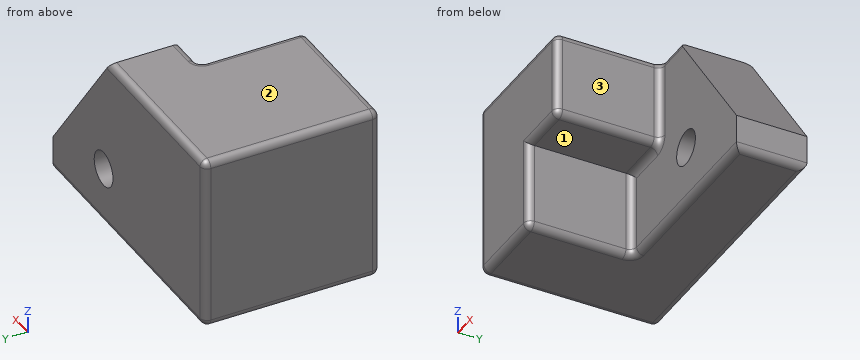
from build123d import *

# Parameters (mm, degrees)
F0_W     = 203.2
F0_H     = 127
F1_DEPTH = 127
F3_DEPTH = 76.2
F4_SIZE2 = 101.6
F4_SIZE  = 76.2
F5_R     = 5.08
F6_R     = 12.6476198181
F7_DEPTH = 78.486


with BuildPart() as f1:
    # F0 (on Front) → F1 (new body)
    with BuildSketch(Plane.XZ):
        Rectangle(F0_W, F0_H)
    extrude(amount=F1_DEPTH)

    # F2 (on face) → F3 (cut)
    with BuildSketch(Plane.XZ.offset(127)):
        Polygon((101.6, 63.5), (0, 63.5), (0, 0), (-38.1, 0), (-38.1, -63.5), (101.6, -63.5), align=None)
    extrude(amount=-F3_DEPTH, mode=Mode.SUBTRACT)

    # F4
    f4_edges = [f1.edges().sort_by_distance(p)[0] for p in [
        (101.6, -25.4, 63.5),
    ]]
    f4_side = f1.faces().sort_by_distance((-21.771429, -52.614286, 63.5))[0]
    chamfer(f4_edges, length=F4_SIZE, length2=F4_SIZE2, reference=f4_side)

    # F5
    f5_edges = [f1.edges().sort_by_distance(p)[0] for p in [
        (0, -88.9, 63.5),
        (-50.8, -127, 63.5),
        (-19.05, -127, 0),
        (0, -127, 31.75),
        (0, -88.9, 0),
        (-38.1, -127, -31.75),
        (-38.1, -88.9, -63.5),
        (-69.85, -127, -63.5),
        (0, -50.8, 31.75),
        (31.75, -50.8, -63.5),
        (-38.1, -50.8, -31.75),
        (0, 0, -63.5),
        (-38.1, 0, 63.5),
        (-101.6, -127, 0),
        (-101.6, -63.5, 63.5),
        (-101.6, 0, 0),
        (101.6, -25.4, -63.5),
        (-101.6, -63.5, -63.5),
        (12.7, -50.8, 63.5),
        (-19.05, -50.8, 0),
    ]]
    fillet(f5_edges, radius=F5_R)

    # F6 (on face) → F7 (cut)
    with BuildSketch(Plane.XZ.offset(50.8)):
        with Locations((33.5065871477, -21.8299999833)):
            Circle(F6_R)
    extrude(amount=-F7_DEPTH, mode=Mode.SUBTRACT)


solid = f1.part
Geometry check sheet. Reference: the model listing, model coordinates, mm. Face numbers are marked on the shaded views. A direction names the side the tool comes from. Round coordinates to 2 decimals unless told otherwise and drop trailing zeros. Write each loop counter-clockwise with the first axis right and the second up, starting at its lowest first coordinate (ties: lowest second). Pieces come first, ordered by that corner, then holes.
Item 1: Go/stop test with flat-tipped pins: pin 1 Ø12 at (x, z) = (80.5, -6) entering from -Y; pin 2 Ø4 at (y, z) = (-111.5, -13.5) entering from +X. Record where each tip stops, or that it passes through.
Determined:
pin 1: stops at y = -50.8
pin 2: stops at x = -38.1
Item 2: Section check C-C (y = -82). Record the boundary of the cut face in (x, z), plus the area to 3 significant figures.
Determined:
outline: (-101.6, -58.42) arc R5.08 ccw to (-96.52, -63.5) - (-43.18, -63.5) arc R5.08 ccw to (-38.1, -58.42) - (-38.1, 0) - (-5.08, 0) arc R5.08 ccw to (0, 5.08) - (0, 58.42) arc R5.08 ccw to (-5.08, 63.5) - (-96.52, 63.5) arc R5.08 ccw to (-101.6, 58.42) - close
area: 10,500 mm2
Item 3: Access from +Z, -Z, +X, -X, +Y, -Y to the whole of each face (thin tool, end or side, straight path). Record for the marked faces 1, 2 and 3.
Determined:
face 1: -Z, +X, -Y
face 2: +Z, +X, -X, +Y, -Y
face 3: +Z, -Z, +X, -Y
Item 4: Section check A-A (y = -27.5). Record the boundary of the cut face in (x, z).
Determined:
outline: (-101.6, -58.42) arc R5.08 ccw to (-96.52, -63.5) - (96.52, -63.5) arc R5.08 ccw to (101.6, -58.42) - (101.6, -38.1) - (25.4, 63.5) - (-96.52, 63.5) arc R5.08 ccw to (-101.6, 58.42) - close; hole circle Ø25.3 at (33.51, -21.83)
Item 5: Section check D-D (z = 41.5). Record the boundary of the cut face in (x, y).
Determined:
outline: (-101.6, -121.92) arc R5.08 ccw to (-96.52, -127) - (-5.08, -127) arc R5.08 ccw to (0, -121.92) - (0, -55.88) arc R5.08 cw to (5.08, -50.8) - (41.9, -50.8) - (41.9, 0) - (-96.52, 0) arc R5.08 ccw to (-101.6, -5.08) - close
Item 6: Section check B-B (z = -21.83). Record the boundary of the cut face in (x, y).
Determined:
outline: (-101.6, -121.92) arc R5.08 ccw to (-96.52, -127) - (-43.18, -127) arc R5.08 ccw to (-38.1, -121.92) - (-38.1, -55.88) arc R5.08 cw to (-33.02, -50.8) - (20.86, -50.8) - (20.86, 0) - (-96.52, 0) arc R5.08 ccw to (-101.6, -5.08) - close; (46.15, -50.8) - (89.4, -50.8) - (89.4, 0) - (46.15, 0) - close
Item 7: Material ranges on line 1 along Y through (x, z) = (38, 19); line 2 along X through (y, z) = (-76, -9.5); line 3 along X through (y, z) = (-32, -21) (3 decimals), recorded low to high.
Determined:
line 1: y = -50.8 to 0
line 2: x = -101.6 to -38.1
line 3: x = -101.6 to 20.886, 46.127 to 88.775
